from build123d import *

# Parameters (mm, degrees)
BOSS_EXTRUDE1_DEPTH     = 6.35
SKETCH2_W               = 63.5
SKETCH2_H               = 10.16
BOSS_EXTRUDE2_DEPTH     = 25.4
SKETCH2_3_W             = 12.7
SKETCH2_3_H             = 23.876
SKETCH2_3_W_2           = 63.5
SKETCH2_3_H_2           = 12.7
CUT_EXTRUDE2_DEPTH      = 72.817261499
CUT_EXTRUDE1_DEPTH      = 27.94
CUT_EXTRUDE1_DEPTH_BACK = 27.94
FILLET1_R               = 2.54
CHAMFER1_SIZE           = 2.54
FILLET2_R               = 2.54
FILLET3_R               = 1.27


with BuildPart() as part:
    # Sketch1 → Boss-Extrude1 (new body)
    with BuildSketch(Plane(origin=(0, 0, 0), x_dir=(1, 0, 0), z_dir=(0, 1, 0))):
        Polygon((-38.1, 37.010512242), (38.1, 37.010512242), (56.060512242, 19.05), (56.060512242, -19.05), (38.1, -37.010512242), (-38.1, -37.010512242), (-56.060512242, -19.05), (-56.060512242, 19.05), align=None)
    extrude(amount=BOSS_EXTRUDE1_DEPTH)

    # Sketch2 → Boss-Extrude2 (add)
    with BuildSketch(Plane(origin=(0, 6.35, 0), x_dir=(1, 0, 0), z_dir=(0, 1, 0))):
        with Locations((0, -6.858)):
            Rectangle(SKETCH2_W, SKETCH2_H)
        with Locations((0, 6.858)):
            Rectangle(SKETCH2_W, SKETCH2_H)
    extrude(amount=BOSS_EXTRUDE2_DEPTH)

    # Sketch2_3 → Cut-Extrude2 (cut, through all)
    with BuildSketch(Plane(origin=(0, 6.35, 0), x_dir=(1, 0, 0), z_dir=(0, 1, 0))):
        with Locations((42.164, 0)):
            Rectangle(SKETCH2_3_W, SKETCH2_3_H)
        with Locations((0, 22.352)):
            Rectangle(SKETCH2_3_W_2, SKETCH2_3_H_2)
        with Locations((-42.164, 0)):
            Rectangle(SKETCH2_3_W, SKETCH2_3_H)
        with Locations((0, -22.352)):
            Rectangle(SKETCH2_3_W_2, SKETCH2_3_H_2)
        Polygon((-35.814, 28.702), (-48.514, 16.002), (-35.814, 16.002), align=None)
        Polygon((35.814, 16.002), (48.514, 16.002), (35.814, 28.702), align=None)
        Polygon((35.810678974, -28.702), (35.810678974, -16.002), (48.514, -16.002), align=None)
        Polygon((-35.814, -16.002), (-48.514, -16.002), (-35.814, -28.702), align=None)
    extrude(amount=-CUT_EXTRUDE2_DEPTH, mode=Mode.SUBTRACT)

    # Sketch3 → Cut-Extrude1 (cut, two sides: drawn at the far end of the back side and taken through both)
    with BuildSketch(Plane(origin=(0, 0, 0), x_dir=(0, 0, -1), z_dir=(1, 0, 0)).offset(-CUT_EXTRUDE1_DEPTH_BACK)):
        with BuildLine():
            Line((-11.938, 31.75), (-4.318, 31.75))
            add(Edge.make_bspline(
                [(-11.938, 6.35), (-6.879920458, 12.89035907), (-4.318, 23.963686989), (-4.318, 31.75)],
                knots=[0, 0, 0, 0, 1, 1, 1, 1], degree=3))
            Line((-11.938, 6.35), (-11.938, 31.75))
        make_face()
        with BuildLine():
            Line((11.938, 6.35), (11.938, 31.75))
            Line((11.938, 31.75), (4.318, 31.75))
            add(Edge.make_bspline(
                [(4.318, 31.75), (4.318, 21.978725734), (6.879920458, 14.349731609), (11.938, 6.35)],
                knots=[0, 0, 0, 0, 1, 1, 1, 1], degree=3))
        make_face()
    extrude(amount=CUT_EXTRUDE1_DEPTH + CUT_EXTRUDE1_DEPTH_BACK, mode=Mode.SUBTRACT)

    # Fillet1
    fillet1_edges = [part.edges().sort_by_distance(p)[0] for p in [
        (-29.845, 31.75, 11.938),
        (29.845, 31.75, -11.938),
        (29.845, 31.75, 11.938),
        (-29.845, 31.75, -11.938),
    ]]
    fillet(fillet1_edges, radius=FILLET1_R)

    # Chamfer1
    chamfer1_edges = [part.edges().sort_by_distance(p)[0] for p in [
        (-47.080256121, 6.35, 28.030256121),
        (0, 6.35, 37.010512242),
        (47.080256121, 6.35, 28.030256121),
        (56.060512242, 6.35, 0),
        (47.080256121, 6.35, -28.030256121),
        (0, 6.35, -37.010512242),
        (-47.080256121, 6.35, -28.030256121),
        (-56.060512242, 6.35, 0),
    ]]
    chamfer(chamfer1_edges, length=CHAMFER1_SIZE)

    # Fillet2
    fillet2_edges = [part.edges().sort_by_distance(p)[0] for p in [
        (-31.75, 6.35, 6.858),
        (31.75, 6.35, 6.858),
        (31.75, 6.35, -6.858),
        (-31.75, 6.35, -6.858),
    ]]
    fillet(fillet2_edges, radius=FILLET2_R)

    # Fillet3
    fillet3_edges = [part.edges().sort_by_distance(p)[0] for p in [
        (48.514, 3.175, -16.002),
        (35.814, 3.175, -16.002),
        (35.814, 3.175, -28.702),
        (35.810678974, 3.175, 28.702),
        (35.810678974, 3.175, 16.002),
        (48.514, 3.175, 16.002),
        (-48.514, 3.175, 16.002),
        (-35.814, 3.175, 16.002),
        (-35.814, 3.175, 28.702),
        (35.814, 3.175, -11.938),
        (48.514, 3.175, -11.938),
        (48.514, 3.175, 11.938),
        (35.814, 3.175, 11.938),
        (-48.514, 3.175, -16.002),
        (-35.814, 3.175, -28.702),
        (-35.814, 3.175, -16.002),
        (31.75, 3.175, 16.002),
        (31.75, 3.175, 28.702),
        (-31.75, 3.175, 28.702),
        (-31.75, 3.175, 16.002),
        (-48.514, 3.175, -11.938),
        (-35.814, 3.175, -11.938),
        (-35.814, 3.175, 11.938),
        (-48.514, 3.175, 11.938),
        (31.75, 3.175, -16.002),
        (-31.75, 3.175, -16.002),
        (-31.75, 3.175, -28.702),
        (31.75, 3.175, -28.702),
    ]]
    fillet(fillet3_edges, radius=FILLET3_R)


solid = part.part
Here's how the part is built. I have some questions about the finished solid (model axes, mm). A direction names the side the tool comes from. Coordinates: 2 decimals unless noted, no trailing zeros. Order: outer loops, then holes, each group sorted by start corner. A loop starts at its lowest first (then second) coordinate and runs counter-clockwise, first axis right, second up. Notation, with made-up numbers: (6.25, 25.5) - (58.25, 25.5) arc R13 cw to (58.25, 37.5) - close; hole circle Ø2 at (21.5, 84). An arc over 180 degrees is marked (long way). Use CSV: the item, a comma, the result in double quotes. Start each with the question number.
1. Please list where these lines run through material, in increasing order: line 1 (X direction, y = 2, z = 3); line 2 (X direction, y = 20, z = 6.5); line 3 (Y direction, x = -14.5, z = -12). Write a range as from..to.
2. Suppose I cut it at C-C on z = -22. List the corners of the cut face in (x, y) for me, then the cut area to 3 significant figures.
3. Suppose I cut it at B-B on x = -40. List the corners of the cut face in (y, z) for me, then the cut area to 3 significant figures.
4. If we mould it in two halves opening along X, with no side actions, what happens to faces 4 (the face through (-56.061, 2, 0)), 5 (the face through (-35.814, 3, -21)), 6 (the face through (0, 19, -1.778)), 7 (the face through (54.81, 5.06, -0.27))? For each: +X half, -X half, draft (parallel to the pull), parting line (faces both ways), or undercut.
5. Suppose I cut it at D-D on y = 2.5. Give the number of separate pieces and of enclosed holes in the cut face, then the cut area to 3 significant figures.
6. Suppose I cut it at A-A on z = -3. List the corners of the cut face in (x, y) for me.
7. I'm going to push flat-ended pins straight in: pin 1 (1.5 mm diameter, centred on y = 5, z = 15, fed in from -X); pin 2 (10 mm diameter, centred on y = 18.5, z = -1.5, fed in from -X); pin 3 (1.9 mm diameter, centred on x = 32, y = 20, fed in from -Z); pin 4 (3 mm diameter, centred on y = 2, z = -20, fed in from +X). Where does each tip first touch, or does it pass through?
8. For faces 1 (the face through (-31.75, 20, -7)), 2 (the face through (0, 3, 16.002)), 3 (the face through (32.514, 7.074, 6.787)), which set-ups out of +Z, -Z, +X, -X, +Y, -Y let a thin tool reach every point of the face, with its end or its side?
Output:
1,line 1,"x = -56.06..-48.51, -35.81..35.81, 48.51..56.06"
1,line 2,"x = -31.75..-27.94, 27.94..31.75"
1,line 3,"y = 0..6.35"
2,outline,"(-53.11, 0) - (-42.52, 0) - (-42.52, 6.35) - (-49.52, 6.35) - (-53.11, 3.81) - close; (-35.81, 0) - (-31.75, 0) - (-31.75, 6.35) - (-35.81, 6.35) - close; (31.75, 0) - (35.81, 0) - (35.81, 6.35) - (31.75, 6.35) - close; (42.52, 0) - (53.11, 0) - (53.11, 3.81) - (49.52, 6.35) - (42.52, 6.35) - close"
2,area,"177 mm2"
3,outline,"(0, -35.11) - (3.81, -35.11) - (6.35, -31.52) - (6.35, -24.52) - (0, -24.52) - close; (0, -16) - (6.35, -16) - (6.35, -11.94) - (0, -11.94) - close; (0, 11.94) - (6.35, 11.94) - (6.35, 16) - (0, 16) - close; (0, 24.52) - (6.35, 24.52) - (6.35, 31.52) - (3.81, 35.11) - (0, 35.11) - close"
3,area,"177 mm2"
4,face 4,"-X half"
4,face 5,"undercut"
4,face 6,"draft"
4,face 7,"+X half"
5,separate pieces,"1"
5,enclosed holes,"8"
5,area,"5,140 mm2"
6,outline,"(-56.06, 0) - (-48.51, 0) - (-48.51, 6.35) - (-53.52, 6.35) - (-56.06, 3.81) - close; (-35.81, 0) - (35.81, 0) - (35.81, 6.35) - (34.29, 6.35) arc R2.54 cw to (31.75, 8.89) - (31.75, 31.75) - (-31.75, 31.75) - (-31.75, 8.89) arc R2.54 cw to (-34.29, 6.35) - (-35.81, 6.35) - close; (48.51, 0) - (56.06, 0) - (56.06, 3.81) - (53.52, 6.35) - (48.51, 6.35) - close"
7,pin 1,"stops at x = -55.62"
7,pin 2,"stops at x = -31.75"
7,pin 3,"stops at z = -11.94"
7,pin 4,"stops at x = 56.06"
8,face 1,"+Z, -Z, -X, +Y"
8,face 2,"+Y, -Y"
8,face 3,"+Z, -Z, +X, +Y"
